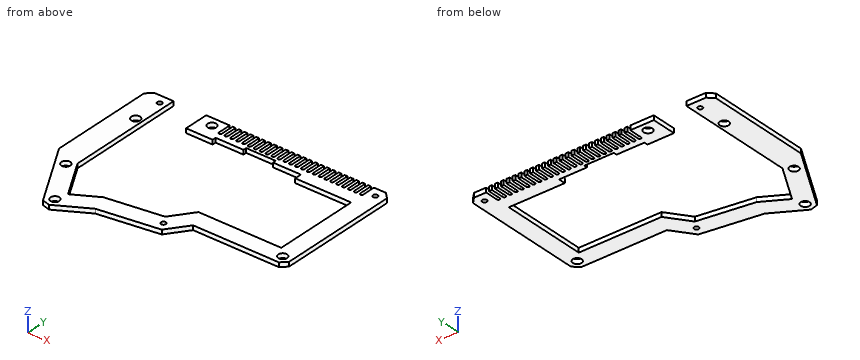
from build123d import *

# Parameters (mm, degrees)
BOSS_EXTRU_2_DEPTH      = 3
ENL_V_MAT_EXTRU_1_DEPTH = 3
ESQUISSE3_R             = 3
ESQUISSE3_R_2           = 1.6
ENL_V_MAT_EXTRU_3_DEPTH = 10


with BuildPart() as part:
    # Esquisse1 → Boss.-Extru.2 (new body)
    with BuildSketch(Plane.XY):
        Polygon((-140.02282508, -78.342807898), (-126.111124489, -102.556497988), (-109.761976756, -93.1463556), (-72.263087593, -87.572177036), (-61.577157206, -72.933633781), (-5.339106961, -72.933633781), (-5.339106961, -14.679643994), (-43.341802282, -14.679643994), (-43.341802282, -9.929307079), (-62.343149943, -9.929307079), (-62.343149943, -7.681038584), (-82.344426674, -7.679926158), (-82.344426674, -9.929307079), (-101.345774335, -9.929307079), (-101.345774335, -12.429484403), (-119.346382005, -12.429484403), (-119.346315028, 4.320852512), (-103.340940531, 4.320852512), (-96.344482292, 4.320852512), (2.832387268, 4.315336518), (6.660893039, 0.486617808), (6.660893039, -81.105206657), (2.832465915, -84.933633781), (-55.479847181, -84.933633781), (-65.531582138, -98.70339941), (-105.747438988, -104.681452952), (-127.216265437, -117.03834868), (-132.440036759, -115.628996046), (-158.478985875, -70.307502815), (-158.478985875, -3.429484403), (-158.478985875, 0.492425388), (-154.65055875, 4.320852512), (-141.52282508, 4.320852512), (-141.52282508, -75.180151251), (-141.52282508, -75.732017442), (-140.889904197, -76.833633309), align=None)
    extrude(amount=BOSS_EXTRU_2_DEPTH)

    # Esquisse2 → Enlèv. mat.-Extru.1 (cut)
    with BuildSketch(Plane.XY.offset(3)):
        with BuildLine():
            Line((-5.339106961, 6.582149677), (-5.339106961, -4.684153384))
            ThreePointArc((-5.339106961, -4.684153384), (-6.339106961, -5.684153384), (-7.339106961, -4.684153384))
            Line((-7.339106961, -4.684153384), (-7.339106961, 6.582149677))
            ThreePointArc((-7.339106961, 6.582149677), (-6.339106961, 7.582149677), (-5.339106961, 6.582149677))
        make_face()
        with BuildLine():
            Line((-9.339106961, 6.582149677), (-9.339106961, -4.684153384))
            ThreePointArc((-9.339106961, -4.684153384), (-10.339106961, -5.684153384), (-11.339106961, -4.684153384))
            Line((-11.339106961, -4.684153384), (-11.339106961, 6.582149677))
            ThreePointArc((-11.339106961, 6.582149677), (-10.339106961, 7.582149677), (-9.339106961, 6.582149677))
        make_face()
        with BuildLine():
            Line((-13.339106961, 6.582149677), (-13.339106961, -4.684153384))
            ThreePointArc((-13.339106961, -4.684153384), (-14.339106961, -5.684153384), (-15.339106961, -4.684153384))
            Line((-15.339106961, -4.684153384), (-15.339106961, 6.582149677))
            ThreePointArc((-15.339106961, 6.582149677), (-14.339106961, 7.582149677), (-13.339106961, 6.582149677))
        make_face()
        with BuildLine():
            Line((-17.339106961, 6.582149677), (-17.339106961, -4.684153384))
            ThreePointArc((-17.339106961, -4.684153384), (-18.339106961, -5.684153384), (-19.339106961, -4.684153384))
            Line((-19.339106961, -4.684153384), (-19.339106961, 6.582149677))
            ThreePointArc((-19.339106961, 6.582149677), (-18.339106961, 7.582149677), (-17.339106961, 6.582149677))
        make_face()
        with BuildLine():
            Line((-21.339106961, 6.582149677), (-21.339106961, -4.684153384))
            ThreePointArc((-21.339106961, -4.684153384), (-22.339106961, -5.684153384), (-23.339106961, -4.684153384))
            Line((-23.339106961, -4.684153384), (-23.339106961, 6.582149677))
            ThreePointArc((-23.339106961, 6.582149677), (-22.339106961, 7.582149677), (-21.339106961, 6.582149677))
        make_face()
        with BuildLine():
            Line((-25.339106961, 6.582149677), (-25.339106961, -4.684153384))
            ThreePointArc((-25.339106961, -4.684153384), (-26.339106961, -5.684153384), (-27.339106961, -4.684153384))
            Line((-27.339106961, -4.684153384), (-27.339106961, 6.582149677))
            ThreePointArc((-27.339106961, 6.582149677), (-26.339106961, 7.582149677), (-25.339106961, 6.582149677))
        make_face()
        with BuildLine():
            Line((-29.339106961, 6.582149677), (-29.339106961, -4.684153384))
            ThreePointArc((-29.339106961, -4.684153384), (-30.339106961, -5.684153384), (-31.339106961, -4.684153384))
            Line((-31.339106961, -4.684153384), (-31.339106961, 6.582149677))
            ThreePointArc((-31.339106961, 6.582149677), (-30.339106961, 7.582149677), (-29.339106961, 6.582149677))
        make_face()
        with BuildLine():
            Line((-33.339106961, 6.582149677), (-33.339106961, -4.684153384))
            ThreePointArc((-33.339106961, -4.684153384), (-34.339106961, -5.684153384), (-35.339106961, -4.684153384))
            Line((-35.339106961, -4.684153384), (-35.339106961, 6.582149677))
            ThreePointArc((-35.339106961, 6.582149677), (-34.339106961, 7.582149677), (-33.339106961, 6.582149677))
        make_face()
        with BuildLine():
            Line((-37.339106961, 6.582149677), (-37.339106961, -4.684153384))
            ThreePointArc((-37.339106961, -4.684153384), (-38.339106961, -5.684153384), (-39.339106961, -4.684153384))
            Line((-39.339106961, -4.684153384), (-39.339106961, 6.582149677))
            ThreePointArc((-39.339106961, 6.582149677), (-38.339106961, 7.582149677), (-37.339106961, 6.582149677))
        make_face()
        with BuildLine():
            Line((-41.339106961, 6.582149677), (-41.339106961, -4.684153384))
            ThreePointArc((-41.339106961, -4.684153384), (-42.339106961, -5.684153384), (-43.339106961, -4.684153384))
            Line((-43.339106961, -4.684153384), (-43.339106961, 6.582149677))
            ThreePointArc((-43.339106961, 6.582149677), (-42.339106961, 7.582149677), (-41.339106961, 6.582149677))
        make_face()
        with BuildLine():
            Line((-45.339106961, 6.582149677), (-45.339106961, -4.684153384))
            ThreePointArc((-45.339106961, -4.684153384), (-46.339106961, -5.684153384), (-47.339106961, -4.684153384))
            Line((-47.339106961, -4.684153384), (-47.339106961, 6.582149677))
            ThreePointArc((-47.339106961, 6.582149677), (-46.339106961, 7.582149677), (-45.339106961, 6.582149677))
        make_face()
        with BuildLine():
            Line((-49.339106961, 6.582149677), (-49.339106961, -4.684153384))
            ThreePointArc((-49.339106961, -4.684153384), (-50.339106961, -5.684153384), (-51.339106961, -4.684153384))
            Line((-51.339106961, -4.684153384), (-51.339106961, 6.582149677))
            ThreePointArc((-51.339106961, 6.582149677), (-50.339106961, 7.582149677), (-49.339106961, 6.582149677))
        make_face()
        with BuildLine():
            Line((-53.339106961, 6.582149677), (-53.339106961, -4.684153384))
            ThreePointArc((-53.339106961, -4.684153384), (-54.339106961, -5.684153384), (-55.339106961, -4.684153384))
            Line((-55.339106961, -4.684153384), (-55.339106961, 6.582149677))
            ThreePointArc((-55.339106961, 6.582149677), (-54.339106961, 7.582149677), (-53.339106961, 6.582149677))
        make_face()
        with BuildLine():
            Line((-57.339106961, 6.582149677), (-57.339106961, -4.684153384))
            ThreePointArc((-57.339106961, -4.684153384), (-58.339106961, -5.684153384), (-59.339106961, -4.684153384))
            Line((-59.339106961, -4.684153384), (-59.339106961, 6.582149677))
            ThreePointArc((-59.339106961, 6.582149677), (-58.339106961, 7.582149677), (-57.339106961, 6.582149677))
        make_face()
        with BuildLine():
            Line((-61.339106961, 6.582149677), (-61.339106961, -4.684153384))
            ThreePointArc((-61.339106961, -4.684153384), (-62.339106961, -5.684153384), (-63.339106961, -4.684153384))
            Line((-63.339106961, -4.684153384), (-63.339106961, 6.582149677))
            ThreePointArc((-63.339106961, 6.582149677), (-62.339106961, 7.582149677), (-61.339106961, 6.582149677))
        make_face()
        with BuildLine():
            Line((-65.339106961, 6.582149677), (-65.339106961, -4.684153384))
            ThreePointArc((-65.339106961, -4.684153384), (-66.339106961, -5.684153384), (-67.339106961, -4.684153384))
            Line((-67.339106961, -4.684153384), (-67.339106961, 6.582149677))
            ThreePointArc((-67.339106961, 6.582149677), (-66.339106961, 7.582149677), (-65.339106961, 6.582149677))
        make_face()
        with BuildLine():
            Line((-69.339106961, 6.582149677), (-69.339106961, -4.684153384))
            ThreePointArc((-69.339106961, -4.684153384), (-70.339106961, -5.684153384), (-71.339106961, -4.684153384))
            Line((-71.339106961, -4.684153384), (-71.339106961, 6.582149677))
            ThreePointArc((-71.339106961, 6.582149677), (-70.339106961, 7.582149677), (-69.339106961, 6.582149677))
        make_face()
        with BuildLine():
            Line((-73.339106961, 6.582149677), (-73.339106961, -4.684153384))
            ThreePointArc((-73.339106961, -4.684153384), (-74.339106961, -5.684153384), (-75.339106961, -4.684153384))
            Line((-75.339106961, -4.684153384), (-75.339106961, 6.582149677))
            ThreePointArc((-75.339106961, 6.582149677), (-74.339106961, 7.582149677), (-73.339106961, 6.582149677))
        make_face()
        with BuildLine():
            Line((-77.339106961, 6.582149677), (-77.339106961, -4.684153384))
            ThreePointArc((-77.339106961, -4.684153384), (-78.339106961, -5.684153384), (-79.339106961, -4.684153384))
            Line((-79.339106961, -4.684153384), (-79.339106961, 6.582149677))
            ThreePointArc((-79.339106961, 6.582149677), (-78.339106961, 7.582149677), (-77.339106961, 6.582149677))
        make_face()
        with BuildLine():
            Line((-81.339106961, 6.582149677), (-81.339106961, -4.684153384))
            ThreePointArc((-81.339106961, -4.684153384), (-82.339106961, -5.684153384), (-83.339106961, -4.684153384))
            Line((-83.339106961, -4.684153384), (-83.339106961, 6.582149677))
            ThreePointArc((-83.339106961, 6.582149677), (-82.339106961, 7.582149677), (-81.339106961, 6.582149677))
        make_face()
        with BuildLine():
            Line((-85.339106961, 6.582149677), (-85.339106961, -4.684153384))
            ThreePointArc((-85.339106961, -4.684153384), (-86.339106961, -5.684153384), (-87.339106961, -4.684153384))
            Line((-87.339106961, -4.684153384), (-87.339106961, 6.582149677))
            ThreePointArc((-87.339106961, 6.582149677), (-86.339106961, 7.582149677), (-85.339106961, 6.582149677))
        make_face()
        with BuildLine():
            Line((-89.339106961, 6.582149677), (-89.339106961, -4.684153384))
            ThreePointArc((-89.339106961, -4.684153384), (-90.339106961, -5.684153384), (-91.339106961, -4.684153384))
            Line((-91.339106961, -4.684153384), (-91.339106961, 6.582149677))
            ThreePointArc((-91.339106961, 6.582149677), (-90.339106961, 7.582149677), (-89.339106961, 6.582149677))
        make_face()
        with BuildLine():
            Line((-93.339106961, 6.582149677), (-93.339106961, -4.684153384))
            ThreePointArc((-93.339106961, -4.684153384), (-94.339106961, -5.684153384), (-95.339106961, -4.684153384))
            Line((-95.339106961, -4.684153384), (-95.339106961, 6.582149677))
            ThreePointArc((-95.339106961, 6.582149677), (-94.339106961, 7.582149677), (-93.339106961, 6.582149677))
        make_face()
        with BuildLine():
            Line((-97.339106961, 6.582149677), (-97.339106961, -4.684153384))
            ThreePointArc((-97.339106961, -4.684153384), (-98.339106961, -5.684153384), (-99.339106961, -4.684153384))
            Line((-99.339106961, -4.684153384), (-99.339106961, 6.582149677))
            ThreePointArc((-99.339106961, 6.582149677), (-98.339106961, 7.582149677), (-97.339106961, 6.582149677))
        make_face()
        with BuildLine():
            Line((-101.339106961, 6.582149677), (-101.339106961, -4.684153384))
            ThreePointArc((-101.339106961, -4.684153384), (-102.339106961, -5.684153384), (-103.339106961, -4.684153384))
            Line((-103.339106961, -4.684153384), (-103.339106961, 6.582149677))
            ThreePointArc((-103.339106961, 6.582149677), (-102.339106961, 7.582149677), (-101.339106961, 6.582149677))
        make_face()
    extrude(amount=-ENL_V_MAT_EXTRU_1_DEPTH, mode=Mode.SUBTRACT)

    # Esquisse3 → Enlèv. mat.-Extru.3 (cut)
    with BuildSketch(Plane.XY):
        with Locations(Location((-110.487646531, -1.678365923, 0), (0, 0, 180))):
            Circle(ESQUISSE3_R)
        with Locations(Location((-146.0923789, -79.822656053, 0), (0, 0, 180))):
            Circle(ESQUISSE3_R)
        with Locations(Location((-128.322250168, -110.752044388, 0), (0, 0, 180))):
            Circle(ESQUISSE3_R)
        with Locations(Location((0.570331496, -78.933633781, 0), (0, 0, 180))):
            Circle(ESQUISSE3_R)
        with Locations(Location((-68.897334865, -93.137788223, 0), (0, 0, 180))):
            Circle(ESQUISSE3_R_2)
        with Locations(Location((-146.02282508, -1.677868186, 0), (0, 0, 180))):
            Circle(ESQUISSE3_R_2)
        with Locations(Location((0.570331496, -1.684542717, 0), (0, 0, 180))):
            Circle(ESQUISSE3_R_2)
        with Locations(Location((-146.02282508, -21.677868186, 0), (0, 0, 180))):
            Circle(ESQUISSE3_R)
    extrude(amount=ENL_V_MAT_EXTRU_3_DEPTH, mode=Mode.SUBTRACT)


solid = part.part
Could you check a few things on this model? Use its own coordinates, in mm. Coordinates: 2 decimals unless noted, no trailing zeros. Loops run counter-clockwise (first coordinate to the right, second up) from the corner with the lowest first, then second, coordinate; pieces in that order, holes last. Notation, with made-up numbers: (89, 15) -> (102, 15) arc R19 cw to (102, 51) -> close; hole circle Ø7 at (-22.75, 0.25). An arc over 180 degrees is marked (long way). Answer in a Markdown table with one row per item.
(1) If I drill on probe 1 along X at (y, z) = (-11.5, 2.5); probe 2 along X at (y, z) = (-39, 2.9); probe 3 along Y at (x, z) = (-52, 0.2), over which ranges is the centre line in solid material (lowest first)?
Results found:
| item | result |
|---|---|
| probe 1 | x = -158.48 to -141.52, -119.35 to -101.35, -43.34 to 6.66 |
| probe 2 | x = -158.48 to -141.52, -5.34 to 6.66 |
| probe 3 | y = -84.93 to -72.93, -9.93 to 4.32 |
(2) Imagine slicing it at C-C (z = 2.25). Give the number of separate pieces and of enclosed holes in the cut face, plus the area to 3 significant figures.
Results found:
| item | result |
|---|---|
| separate pieces | 1 |
| enclosed holes | 8 |
| area | 5,630 mm^2 |
(3) Will these pins go through, and if not, where does the flat tip stop? pin 1 Ø0.6 at (x, z) = (-16.5, 2) entering from +Y; pin 2 Ø1.5 at (x, z) = (-76, 1) entering from -Y; pin 3 Ø0.9 at (x, z) = (-21.5, 1.5) entering from -Y.
Results found:
| item | result |
|---|---|
| pin 1 | stops at y = 4.32 |
| pin 2 | stops at y = -100.37 |
| pin 3 | stops at y = -84.93 |
(4) Imagine slicing it at B-B (x = -117). List the corners of the cut face in (y, z) for me, plus the area to 3 significant figures.
Results found:
| item | result |
|---|---|
| outline | (-111.16, 0) -> (-97.31, 0) -> (-97.31, 3) -> (-111.16, 3) -> close; (-12.43, 0) -> (4.32, 0) -> (4.32, 3) -> (-12.43, 3) -> close |
| area | 91.8 mm^2 |
(5) Imagine slicing it at A-A (y = -66.5). List the corners of the cut face in (x, z) for me.
Results found:
| item | result |
|---|---|
| outline | (-158.48, 0) -> (-141.52, 0) -> (-141.52, 3) -> (-158.48, 3) -> close; (-5.34, 0) -> (6.66, 0) -> (6.66, 3) -> (-5.34, 3) -> close |
